```python
from build123d import *

# Parameters (mm, degrees)
F1_DEPTH      = 203.2
F3_DEPTH      = 38.101
F3_DEPTH_BACK = 38.101


with BuildPart() as f1:
    # F0 (on Front) → F1 (new body)
    with BuildSketch(Plane.XZ):
        with BuildLine():
            ThreePointArc((25.4, 34.925), (24.4700640303, 37.1700640303), (22.225, 38.1))
            Line((22.225, 38.1), (-22.225, 38.1))
            ThreePointArc((-22.225, 38.1), (-24.4700640303, 37.1700640303), (-25.4, 34.925))
            Line((-25.4, 34.925), (-25.4, -34.925))
            ThreePointArc((-25.4, -34.925), (-24.4700640303, -37.1700640303), (-22.225, -38.1))
            Line((-22.225, -38.1), (22.225, -38.1))
            ThreePointArc((22.225, -38.1), (24.4700640303, -37.1700640303), (25.4, -34.925))
            Line((25.4, -34.925), (25.4, 34.925))
        make_face()
        with BuildLine():
            Line((-19.05, 34.925), (19.05, 34.925))
            ThreePointArc((19.05, 34.925), (21.2950640303, 33.9950640303), (22.225, 31.75))
            Line((22.225, 31.75), (22.225, -31.75))
            ThreePointArc((22.225, -31.75), (21.2950640303, -33.9950640303), (19.05, -34.925))
            Line((19.05, -34.925), (-19.05, -34.925))
            ThreePointArc((-19.05, -34.925), (-21.2950640303, -33.9950640303), (-22.225, -31.75))
            Line((-22.225, -31.75), (-22.225, 31.75))
            ThreePointArc((-22.225, 31.75), (-21.2950640303, 33.9950640303), (-19.05, 34.925))
        make_face(mode=Mode.SUBTRACT)
    extrude(amount=F1_DEPTH)

    # F2 (on Top) → F3 (cut, two sides)
    with BuildSketch(Plane.XY) as f3_sk:
        Polygon((-25.4, -203.2), (25.4, -203.2), (-25.4, -183.6997070202), align=None)
    extrude(amount=-F3_DEPTH, mode=Mode.SUBTRACT)
    extrude(f3_sk.sketch, amount=F3_DEPTH_BACK, mode=Mode.SUBTRACT)


solid = f1.part
```
Build history of the part. All positions in model axes, mm. A direction names the side the tool comes from. Round coordinates to 2 decimals unless told otherwise and drop trailing zeros. Write each loop counter-clockwise with the first axis right and the second up, starting at its lowest first coordinate (ties: lowest second). Pieces come first, ordered by that corner, then holes.
1) Drill centre lines: probe 1 along Z at (x, y) = (-19, -59) (3 decimals); probe 2 along X at (y, z) = (-169.5, 32); probe 3 along X at (y, z) = (-188.5, -9.5) (3 decimals). Where is each one in solid material? Low to high.
2) Band-saw the part on D-D, the plane y = -189. List the corners of the cut face in (x, z) (3 decimals).
3) Band-saw the part on C-C, the plane y = -115. List the corners of the cut face in (x, z) (3 decimals).
4) Band-saw the part on A-A, the plane z = -20. List the corners of the cut face in (x, y) (3 decimals), and give its area (3 significant figures).
5) Band-saw the part on B-B, the plane x = -6. List the corners of the cut face in (y, z) (3 decimals), and give its area (3 significant figures).
6) Mould opens along X. For faces 1 (the flat face through (25.4, -100, 0)), 2 (the flat face through (0, -99, 34.925)), 3 (the flat face through (-23, 0, 3)) say: +X half, -X half, draft (parallel to the pull), parting line (faces both ways), or undercut.
7) 3-axis set-ups, long thin cutter, end or side, ignore diameter. For faces 4 (the flat face through (-22.225, -91, 0)), 5 (the flat face through (22.696, -202.162, -3)): which of +Z, -Z, +X, -X, +Y, -Y reach the whole face in a straight line?
Ans:
1. probe 1: z = -38.1 to -34.925, 34.925 to 38.1
1. probe 2: x = -25.4 to -22.22, 22.22 to 25.4
1. probe 3: x = 22.225 to 25.4
2. outline: (-11.592, -38.1) - (22.225, -38.1) arc R3.175 ccw to (25.4, -34.925) - (25.4, 34.925) arc R3.175 ccw to (22.225, 38.1) - (-11.592, 38.1) - (-11.592, 34.925) - (19.05, 34.925) arc R3.175 cw to (22.225, 31.75) - (22.225, -31.75) arc R3.175 cw to (19.05, -34.925) - (-11.592, -34.925) - close
3. outline: (-25.4, -34.925) arc R3.175 ccw to (-22.225, -38.1) - (22.225, -38.1) arc R3.175 ccw to (25.4, -34.925) - (25.4, 34.925) arc R3.175 ccw to (22.225, 38.1) - (-22.225, 38.1) arc R3.175 ccw to (-25.4, 34.925) - close; hole (-22.225, -31.75) arc R3.175 ccw to (-19.05, -34.925) - (19.05, -34.925) arc R3.175 ccw to (22.225, -31.75) - (22.225, 31.75) arc R3.175 ccw to (19.05, 34.925) - (-19.05, 34.925) arc R3.175 ccw to (-22.225, 31.75) - close
4. outline: (-25.4, -183.7) - (-22.225, -184.918) - (-22.225, 0) - (-25.4, 0) - close; (22.225, -201.981) - (25.4, -203.2) - (25.4, 0) - (22.225, 0) - close
4. area: 1,230 mm2
5. outline: (-191.147, -38.1) - (0, -38.1) - (0, -34.925) - (-191.147, -34.925) - close; (-191.147, 34.925) - (0, 34.925) - (0, 38.1) - (-191.147, 38.1) - close
5. area: 1,210 mm2
6. face 1: +X half
6. face 2: undercut
6. face 3: draft
7. face 4: +Y, -Y
7. face 5: +Z, -Z, -X, -Y
